Check sheet for the drawn part. Datum: minimum x, y, z corner. Units: mm. A direction names the side the tool comes from. Coordinates: 2 decimals unless noted, no trailing zeros. Write each loop counter-clockwise with the first axis right and the second up, starting at its lowest first coordinate (ties: lowest second). Pieces come first, ordered by that corner, then holes. Notation, with made-up numbers: M -38.5,50 L -1.5,50 A33 cw -1.5,83 Z; hole C 62,41 d5. An arc over 180 degrees is marked long. Answer in a Markdown table with one row per item.
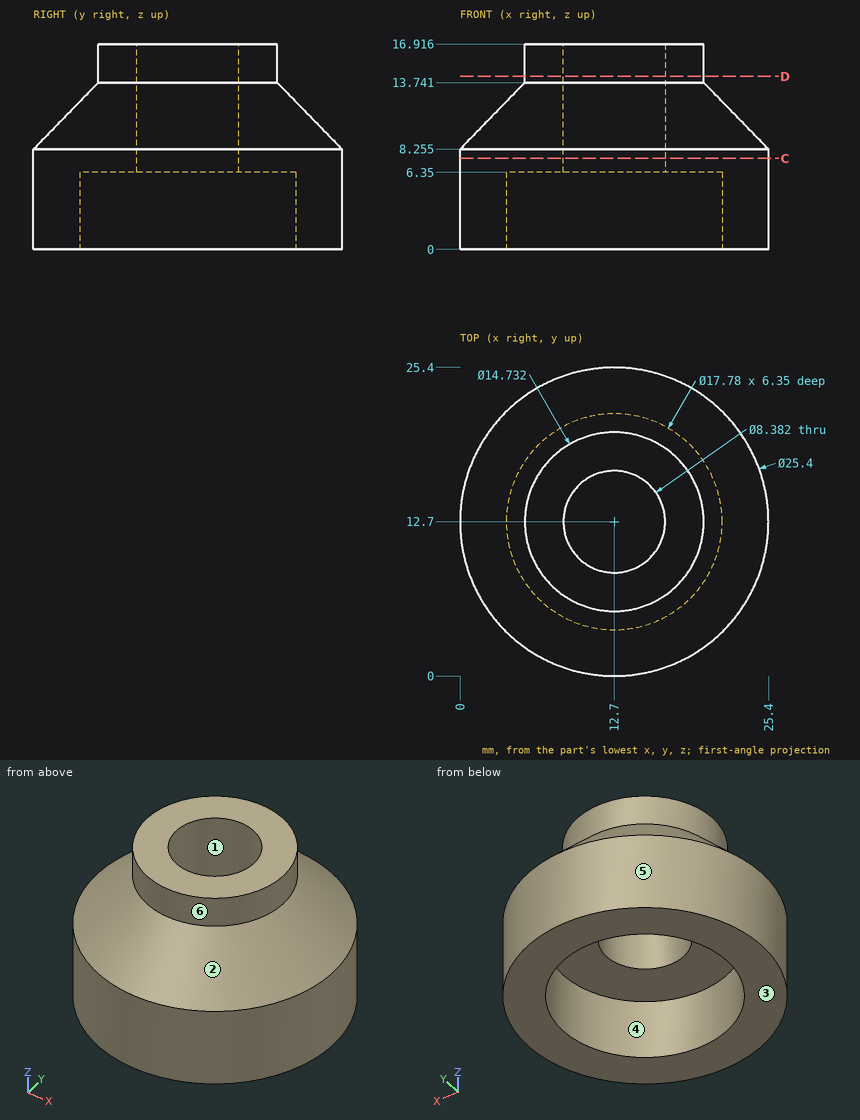
1) Release check for a two-part mould opening along X. For the marked faces 1, 2 and 3 record: +X half, -X half, draft (parallel to the pull), parting line (faces both ways), or undercut.
Response values:
| item | result |
|---|---|
| face 1 | undercut |
| face 2 | parting line |
| face 3 | draft |
2) Tool access check on the marked faces 4, 5 and 6. Record the directions out of +Z, -Z, +X, -X, +Y, -Y that give a thin tool (end or side, any length) a straight path to the whole face; none if there is none.
Response values:
| item | result |
|---|---|
| face 4 | -Z |
| face 5 | +Z, -Z |
| face 6 | +Z |
3) Sectioned sample at D-D (z = 14.25). Record the cut outline in (x, y), then the cut area to 3 significant figures.
Response values:
| item | result |
|---|---|
| outline | C 12.7,12.7 d14.73; hole C 12.7,12.7 d8.38 |
| area | 115 mm² |
4) Sectioned sample at C-C (z = 7.5). Record the cut outline in (x, y).
Response values:
| item | result |
|---|---|
| outline | C 12.7,12.7 d25.4; hole C 12.7,12.7 d8.38 |
5) Thickness scan on L1, parallel to Y at x = 12.7, z = 5; L2, parallel to Z at x = 11.75, y = 19.25; L3, parallel to Y at x = 12.7, z = 12.5 (1 decimal). Record the ranges inside material, lowest first. Write a range as [from, to].
Response values:
| item | result |
|---|---|
| L1 | y = [0, 3.81], [21.59, 25.4] |
| L2 | z = [6.35, 16.92] |
| L3 | y = [4.1, 8.5], [16.9, 21.3] |
6) Depth check by flat-ended pin: pin 1 (6.5 mm diameter, centred on x = 12.7, y = 12.7, fed in from -Z); pin 2 (5 mm diameter, centred on y = 5, z = 8.5, fed in from +X); pin 3 (1 mm diameter, centred on x = 12.5, z = 12.5, fed in from +Y); pin 4 (2 mm diameter, centred on x = 16.5, z = 10, fed in from +Y) (1 decimal). Enter the tip coordinate at first touch or a pass-through.
Response values:
| item | result |
|---|---|
| pin 1 | passes through |
| pin 2 | stops at x = 24.28 |
| pin 3 | stops at y = 21.76 |
| pin 4 | stops at y = 24.1 |
